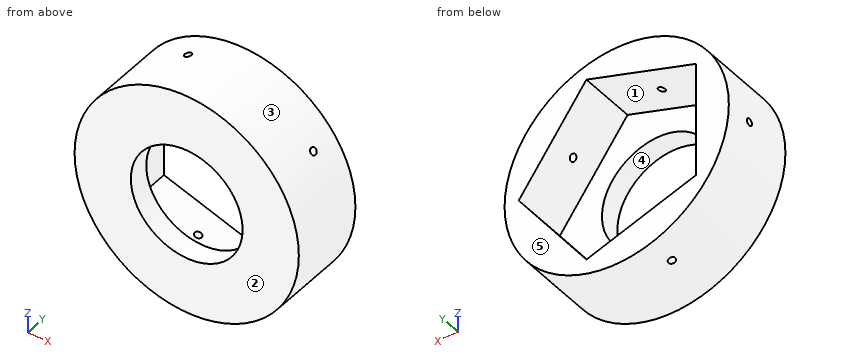
from build123d import *

# Parameters (mm, degrees)
SKETCH1_R                = 69.57983352
SKETCH1_R_2              = 39.6875
BOSS_EXTRUDE1_DEPTH      = 15
SKETCH2_R                = 79.57983352
SKETCH2_R_2              = 69.57983352
BOSS_EXTRUDE2_DEPTH      = 40
BOSS_EXTRUDE2_DEPTH_BACK = 15
BOSS_EXTRUDE3_DEPTH      = 40
SKETCH4_R                = 2.5
CUT_EXTRUDE1_DEPTH       = 44.985172419
CIRPATTERN1_COUNT        = 5


with BuildPart() as part:
    # Sketch1 → Boss-Extrude1 (new body)
    with BuildSketch(Plane(origin=(0, 0, 0), x_dir=(1, 0, 0), z_dir=(0, 1, 0))):
        Circle(SKETCH1_R)
        Circle(SKETCH1_R_2, mode=Mode.SUBTRACT)
    extrude(amount=BOSS_EXTRUDE1_DEPTH)

    # Sketch2 → Boss-Extrude2 (add, two sides)
    with BuildSketch(Plane(origin=(0, 15, 0), x_dir=(1, 0, 0), z_dir=(0, 1, 0))) as boss_extrude2_sk:
        Circle(SKETCH2_R)
        Circle(SKETCH2_R_2, mode=Mode.SUBTRACT)
    extrude(amount=BOSS_EXTRUDE2_DEPTH)
    extrude(boss_extrude2_sk.sketch, amount=-BOSS_EXTRUDE2_DEPTH_BACK)

    # Sketch3 → Boss-Extrude3 (add)
    with BuildSketch(Plane(origin=(0, 15, 0), x_dir=(1, 0, 0), z_dir=(0, 1, 0))):
        with BuildLine():
            ThreePointArc((21.501351023, -66.174354072), (56.291267783, -40.898), (69.57983352, 0))
            Line((69.57983352, 0), (21.501351023, -66.174354072))
        make_face()
        with BuildLine():
            Line((21.501351023, 66.174354072), (69.57983352, 0))
            ThreePointArc((69.57983352, 0), (56.291267783, 40.898), (21.501351023, 66.174354072))
        make_face()
        with BuildLine():
            Line((-56.291267783, 40.898), (21.501351023, 66.174354072))
            ThreePointArc((21.501351023, 66.174354072), (-21.501351023, 66.174354072), (-56.291267783, 40.898))
        make_face()
        with BuildLine():
            ThreePointArc((-56.291267783, -40.898), (-21.501351023, -66.174354072), (21.501351023, -66.174354072))
            Line((21.501351023, -66.174354072), (-56.291267783, -40.898))
        make_face()
        with BuildLine():
            Line((-56.291267783, -40.898), (-56.291267783, 40.898))
            ThreePointArc((-56.291267783, 40.898), (-69.57983352, 0), (-56.291267783, -40.898))
        make_face()
    extrude(amount=BOSS_EXTRUDE3_DEPTH)

    # Sketch4 → Cut-Extrude1 (cut, through all)
    with BuildSketch(Plane(origin=(-17.39495838, 0, -53.536177036), x_dir=(0.951056516, 0, -0.309016994), z_dir=(0.309016994, 0, 0.951056516))):
        with Locations((0, 35)):
            Circle(SKETCH4_R)
    cut_extrude1 = extrude(amount=-CUT_EXTRUDE1_DEPTH, mode=Mode.SUBTRACT)

    # CirPattern1: Cut-Extrude1 ×5 about axis
    cirpattern1_axis = Axis((0, -225.085759711, 0), (0, 1, 0))
    for i in range(1, CIRPATTERN1_COUNT):
        add(cut_extrude1.rotate(cirpattern1_axis, i * 360 / CIRPATTERN1_COUNT), mode=Mode.SUBTRACT)


solid = part.part
Model file for the job. Use its own axes, mm. Face numbers are marked on the shaded views. A direction names the side the tool comes from. Coordinates: 2 decimals unless noted, no trailing zeros. Order: outer loops, then holes, each group sorted by start corner. A loop starts at its lowest first (then second) coordinate and runs counter-clockwise, first axis right, second up. Notation, with made-up numbers: (31, -20.75) -> (38, -20.75) arc R21 ccw to (38, -15.75) -> close; hole circle Ø3 at (18, 40.5). An arc over 180 degrees is marked (long way). Return JSON: item names as keys, results as strings. Group by question number.
Item 1: Wall check: line 1 along Y through (x, z) = (49.5, 36); line 2 along X through (y, z) = (5, 0). Give the ranges that are in metal, low to high. Write a range as [from, to].
Item 2: Flat gauge pins, fed straight in: P1, Ø4, axis at x = 51, y = 6, coming from the +Z side; P2, Ø6, axis at y = 17, z = -5, coming from the -X side; P3, Ø6, axis at x = -43.5, y = 45, coming from the +Z side. Where does each tip first touch, or does it go through?
Item 3: Saw through at B-B on z = -23. Write the cut outline in (x, y), then the cut area to 3 significant figures.
Item 4: Saw through at C-C on y = 35. Write the cut outline in (x, z).
Item 5: Tool access for the marked faces 1 and 2: list every direction of +Z, -Z, +X, -X, +Y, -Y with a clear straight run to the whole face (end or side of a thin tool).
Item 6: Saw through at A-A on x = -10.5. Write the cut outline in (y, z), then the cut area to 3 significant figures.
Item 7: Pull direction X, two halves, no side cores. Call the marked faces 3, 4 and 5: pulls with the +X half, pulls with the -X half, needs draft (parallel to the pull), parting line crosses it, or undercut.
Item 8: Saw through at D-D on y = 20. Write the cut outline in (x, z), then the cut area to 3 significant figures.
Values found:
{
 "1": {"line 1": "y = [0, 32.5], [37.5, 55]", "line 2": "x = [-79.58, -39.69], [39.69, 79.58]"},
 "2": {"P1": "stops at z = 62.71", "P2": "stops at x = -79.55", "P3": "stops at z = 68.5"},
 "3": {"outline": "(-76.18, 0) -> (-32.34, 0) -> (-32.34, 15) -> (-56.29, 15) -> (-56.29, 55) -> (-76.18, 55) -> close; (32.34, 0) -> (76.18, 0) -> (76.18, 55) -> (52.87, 55) -> (52.87, 15) -> (32.34, 15) -> close", "area": "3,040 mm2"},
 "4": {"outline": "(-79.54, -2.5) arc R79.58 ccw to (-26.96, -74.88) -> (-19.77, -52.76) -> (-56.29, -40.9) -> (-56.29, -2.5) -> close; (-79.54, 2.5) -> (-56.29, 2.5) -> (-56.29, 40.9) -> (-19.77, 52.76) -> (-26.96, 74.88) arc R79.58 ccw to start; (-22.2, -76.42) arc R79.58 ccw to (62.88, -48.78) -> (44.07, -35.11) -> (21.5, -66.17) -> (-15.02, -54.31) -> close; (-22.2, 76.42) -> (-15.02, 54.31) -> (21.5, 66.17) -> (44.07, 35.11) -> (62.88, 48.78) arc R79.58 ccw to start; (47.01, -31.06) -> (65.82, -44.73) arc R79.58 ccw to (65.82, 44.73) -> (47.01, 31.06) -> (69.58, 0) -> close"},
 "5": {"face 1": "+Y", "face 2": "+Z, -Z, +X, -X, -Y"},
 "6": {"outline": "(0, -78.88) -> (55, -78.88) -> (55, -55.78) -> (15, -55.78) -> (15, -38.27) -> (0, -38.27) -> close; (0, 38.27) -> (15, 38.27) -> (15, 55.78) -> (55, 55.78) -> (55, 78.88) -> (0, 78.88) -> close", "area": "3,070 mm2"},
 "7": {"face 3": "parting line crosses it", "face 4": "undercut", "face 5": "needs draft"},
 "8": {"outline": "circle Ø159.16 at (0, 0); hole (-56.29, -40.9) -> (21.5, -66.17) -> (69.58, 0) -> (21.5, 66.17) -> (-56.29, 40.9) -> close", "area": "8,380 mm2"}
}
